```python
from build123d import *

# Parameters (mm, degrees)
SKETCH1_W                      = 150
SKETCH1_H                      = 30
BOSS_EXTRUDE1_DEPTH            = 5
F_6_0MM_DOWEL_HOLE1_AT_2_COUNT = 2
F_6_0MM_DOWEL_HOLE1_AT_2_PITCH = 37.5
F_4_0MM_DOWEL_HOLE1_AT_2_COUNT = 2
F_4_0MM_DOWEL_HOLE1_AT_2_PITCH = 37.5
F_12_0MM_DOWEL_HOLE2_D         = 12
F_12_0MM_DOWEL_HOLE2_DEPTH     = 25
F_12_0MM_DOWEL_HOLE2_TIP       = 3.605163714
SKETCH30_W                     = 150
SKETCH30_H                     = 15
CUT_EXTRUDE1_DEPTH             = 10
F_12_0MM_DOWEL_HOLE3_D         = 12
F_12_0MM_DOWEL_HOLE3_DEPTH     = 12.75
F_12_0MM_DOWEL_HOLE3_TIP       = 3.605163714


with BuildPart() as part:
    # Sketch1 → Boss-Extrude1 (new body)
    with BuildSketch(Plane.XY):
        with Locations((18.189254194, 3.553058878)):
            Rectangle(SKETCH1_W, SKETCH1_H)
    extrude(amount=BOSS_EXTRUDE1_DEPTH)

    # Sketch4 → Ø6.0mm Dowel Hole1 (revolve, cut)
    with BuildSketch(Plane(origin=(55.689254194, 3.553058878, 5), x_dir=(0, -1, 0), z_dir=(1, 0, 0))):
        Polygon((0, 0), (0, 26.802581857), (3, 25), (3, 0), align=None)
    f_6_0mm_dowel_hole1 = revolve(axis=Axis((55.689254194, 3.553058878, 11.35), (0, 0, -1)), mode=Mode.SUBTRACT)

    # Ø6.0mm Dowel Hole1 at 2: Ø6.0mm Dowel Hole1 ×2
    with Locations(*[(-i * F_6_0MM_DOWEL_HOLE1_AT_2_PITCH, 0, 0) for i in range(1, F_6_0MM_DOWEL_HOLE1_AT_2_COUNT)]):
        add(f_6_0mm_dowel_hole1, mode=Mode.SUBTRACT)

    # Mirror1: Ø6.0mm Dowel Hole1 across plane
    add(f_6_0mm_dowel_hole1.mirror(Plane.ZY.offset(-18.189254194)), mode=Mode.SUBTRACT)

    # Mirror1 copy 1 sketch → Mirror1 copy 1 (revolve, cut)
    with BuildSketch(Plane(origin=(18.189254194, 3.553058878, 5), x_dir=(0, -1, 0), z_dir=(-1, 0, 0))):
        Polygon((0, 0), (0, -26.802581857), (3, -25), (3, 0), align=None)
    revolve(axis=Axis((18.189254194, 3.553058878, 11.35), (0, 0, 1)), mode=Mode.SUBTRACT)

    # Sketch6 → Ø4.0mm Dowel Hole1 (revolve, cut)
    with BuildSketch(Plane(origin=(74.439254194, 11.053058878, 5), x_dir=(0, -1, 0), z_dir=(1, 0, 0))):
        Polygon((0, 0), (0, 26.201721238), (2, 25), (2, 0), align=None)
    f_4_0mm_dowel_hole1 = revolve(axis=Axis((74.439254194, 11.053058878, 11.35), (0, 0, -1)), mode=Mode.SUBTRACT)

    # Ø4.0mm Dowel Hole1 at 2: Ø4.0mm Dowel Hole1 ×2
    with Locations(*[(-i * F_4_0MM_DOWEL_HOLE1_AT_2_PITCH, 0, 0) for i in range(1, F_4_0MM_DOWEL_HOLE1_AT_2_COUNT)]):
        add(f_4_0mm_dowel_hole1, mode=Mode.SUBTRACT)

    # Mirror2: Ø4.0mm Dowel Hole1 across plane
    add(f_4_0mm_dowel_hole1.mirror(Plane.ZX.offset(3.553058878)), mode=Mode.SUBTRACT)

    # Mirror2 copy 1 sketch → Mirror2 copy 1 (revolve, cut)
    with BuildSketch(Plane(origin=(36.939254194, -3.946941122, 5), x_dir=(0, 1, 0), z_dir=(1, 0, 0))):
        Polygon((0, 0), (0, -26.201721238), (2, -25), (2, 0), align=None)
    revolve(axis=Axis((36.939254194, -3.946941122, 11.35), (0, 0, 1)), mode=Mode.SUBTRACT)

    # Mirror3: Ø4.0mm Dowel Hole1 across plane
    add(f_4_0mm_dowel_hole1.mirror(Plane.ZY.offset(-18.189254194)), mode=Mode.SUBTRACT)

    # Mirror3 copy 1 sketch → Mirror3 copy 1 (revolve, cut)
    with BuildSketch(Plane(origin=(-38.060745806, -3.946941122, 5), x_dir=(0, 1, 0), z_dir=(-1, 0, 0))):
        Polygon((0, 0), (0, 26.201721238), (2, 25), (2, 0), align=None)
    revolve(axis=Axis((-38.060745806, -3.946941122, 11.35), (0, 0, -1)), mode=Mode.SUBTRACT)

    # Mirror3 copy 2 sketch → Mirror3 copy 2 (revolve, cut)
    with BuildSketch(Plane(origin=(-0.560745806, -3.946941122, 5), x_dir=(0, 1, 0), z_dir=(-1, 0, 0))):
        Polygon((0, 0), (0, 26.201721238), (2, 25), (2, 0), align=None)
    revolve(axis=Axis((-0.560745806, -3.946941122, 11.35), (0, 0, -1)), mode=Mode.SUBTRACT)

    # Mirror3 copy 3 sketch → Mirror3 copy 3 (revolve, cut)
    with BuildSketch(Plane(origin=(-0.560745806, 11.053058878, 5), x_dir=(0, -1, 0), z_dir=(-1, 0, 0))):
        Polygon((0, 0), (0, -26.201721238), (2, -25), (2, 0), align=None)
    revolve(axis=Axis((-0.560745806, 11.053058878, 11.35), (0, 0, 1)), mode=Mode.SUBTRACT)

    # Sketch23 → Ø3.0mm Dowel Hole2 (revolve, cut)
    with BuildSketch(Plane(origin=(-47.435745806, -3.946941122, 5), x_dir=(0, -1, 0), z_dir=(1, 0, 0))):
        Polygon((0, 0), (0, 25.901290929), (1.5, 25), (1.5, 0), align=None)
    f_3_0mm_dowel_hole2 = revolve(axis=Axis((-47.435745806, -3.946941122, 11.35), (0, 0, -1)), mode=Mode.SUBTRACT)

    # Mirror5: Ø3.0mm Dowel Hole2 across plane
    add(f_3_0mm_dowel_hole2.mirror(Plane.ZY.offset(-18.189254194)), mode=Mode.SUBTRACT)

    # Ø12.0mm Dowel Hole2
    with Locations(Plane(origin=(26.189254194, 3.553058878, 5), x_dir=(1, 0, 0), z_dir=(0, 0, 1))):
        with Locations((0, 0)):
            Hole(F_12_0MM_DOWEL_HOLE2_D / 2, depth=F_12_0MM_DOWEL_HOLE2_DEPTH)
            with Locations((0, 0, -(F_12_0MM_DOWEL_HOLE2_DEPTH + F_12_0MM_DOWEL_HOLE2_TIP / 2))):  # 118° drill point
                Cone(0, F_12_0MM_DOWEL_HOLE2_D / 2, F_12_0MM_DOWEL_HOLE2_TIP, mode=Mode.SUBTRACT)

    # Sketch30 → Cut-Extrude1 (cut)
    with BuildSketch(Plane.XY.offset(5)):
        with Locations((18.189254194, 11.053058878)):
            Rectangle(SKETCH30_W, SKETCH30_H)
    extrude(amount=-CUT_EXTRUDE1_DEPTH, mode=Mode.SUBTRACT)

    # Ø12.0mm Dowel Hole3
    with Locations(Plane.XY.offset(5)):
        with Locations((63.689254194, 3.553058878), (-27.310745806, 3.553058878)):
            Hole(F_12_0MM_DOWEL_HOLE3_D / 2, depth=F_12_0MM_DOWEL_HOLE3_DEPTH)
            with Locations((0, 0, -(F_12_0MM_DOWEL_HOLE3_DEPTH + F_12_0MM_DOWEL_HOLE3_TIP / 2))):  # 118° drill point
                Cone(0, F_12_0MM_DOWEL_HOLE3_D / 2, F_12_0MM_DOWEL_HOLE3_TIP, mode=Mode.SUBTRACT)


solid = part.part
```
Build history of the part. All positions in model axes, mm. Coordinates: 2 decimals unless noted, no trailing zeros. Order: outer loops, then holes, each group sorted by start corner. A loop starts at its lowest first (then second) coordinate and runs counter-clockwise, first axis right, second up. Notation, with made-up numbers: (23.25, 8.25) -> (32.25, 8.25) arc R7 ccw to (32.25, 13.25) -> close; hole circle Ø6 at (77, 35). An arc over 180 degrees is marked (long way). Answer in a Markdown table with one row per item. Add a question column.
Q1. Wall check: line 1 along X through (y, z) = (-0.5, 3.9); line 2 along X through (y, z) = (0, 4.75); line 3 along Y through (x, z) = (-1, 2.7). Give the ranges that are in metal, low to high. Write a range as [from, to].
Q2. Band-saw the part on D-D, the plane x = -30.5. List the corners of the cut face in (y, z), then the cut area to 3 significant figures.
Q3. Band-saw the part on C-C, the plane x = 19. List the corners of the cut face in (y, z), then the cut area to 3 significant figures.
Q4. Band-saw the part on B-B, the plane y = -4. List the corners of the cut face in (x, z), then the cut area to 3 significant figures.
Q5. Band-saw the part on A-A, the plane z = 2.35. List the corners of the cut face in (x, y), then the cut area to 3 significant figures.
Q6. Mould opens along Y. For faces 1 (the face through (17, -4, 5)), 2 (the face through (-0.473, -5.945, 2.535)), 3 (the face through (17, -11.447, 2)), 4 (the face through (-39.835, -3.024, 2.535)) say: +Y half, -Y half, draft (parallel to the pull), parting line (faces both ways), or undercut.
Q7. Drop a flat-ended pin along its axis: pin 1 (3 mm diameter, centred on x = -0.56, y = -3.95, fed in from +Z). Give the stop position or say it passes through.
Answers follow:
| question | item | result |
|---|---|---|
| 1 | line 1 | [-56.81, -31.73], [-22.89, 21.77], [30.61, 59.27], [68.11, 93.19] |
| 1 | line 2 | [-56.81, -32.15], [-22.48, 21.35], [31.02, 58.85], [68.52, 93.19] |
| 1 | line 3 | [-11.45, -5.9], [-2, 3.55] |
| 2 | outline | (-11.45, 0) -> (-1.53, 0) -> (-1.53, 5) -> (-11.45, 5) -> close |
| 2 | area | 49.6 mm^2 |
| 3 | outline | (-11.45, 0) -> (0.66, 0) -> (0.66, 5) -> (-11.45, 5) -> close |
| 3 | area | 60.6 mm^2 |
| 4 | outline | (-56.81, 0) -> (-48.93, 0) -> (-48.93, 5) -> (-56.81, 5) -> close; (-45.94, 0) -> (-40.06, 0) -> (-40.06, 5) -> (-45.94, 5) -> close; (-36.06, 0) -> (-2.56, 0) -> (-2.56, 5) -> (-36.06, 5) -> close; (1.44, 0) -> (34.94, 0) -> (34.94, 5) -> (1.44, 5) -> close; (38.94, 0) -> (72.44, 0) -> (72.44, 5) -> (38.94, 5) -> close; (76.44, 0) -> (82.32, 0) -> (82.32, 5) -> (76.44, 5) -> close; (85.31, 0) -> (93.19, 0) -> (93.19, 5) -> (85.31, 5) -> close |
| 4 | area | 640 mm^2 |
| 5 | outline | (-56.81, -11.45) -> (93.19, -11.45) -> (93.19, 3.55) -> (69.69, 3.55) arc R6 cw to (58, 1.64) arc R3 cw to (52.69, 3.55) -> (32.19, 3.55) arc R6 cw to (20.5, 1.64) arc R3 cw to (15.19, 3.55) -> (-16.31, 3.55) arc R3 cw to (-21.62, 1.64) arc R6 cw to (-33.31, 3.55) -> (-56.81, 3.55) -> close; hole circle Ø3 at (-47.44, -3.95); hole circle Ø4 at (-38.06, -3.95); hole circle Ø4 at (-0.56, -3.95); hole circle Ø4 at (36.94, -3.95); hole circle Ø4 at (74.44, -3.95); hole circle Ø3 at (83.81, -3.95) |
| 5 | area | 1,980 mm^2 |
| 6 | face 1 | draft |
| 6 | face 2 | undercut |
| 6 | face 3 | -Y half |
| 6 | face 4 | undercut |
| 7 | pin 1 | through |
